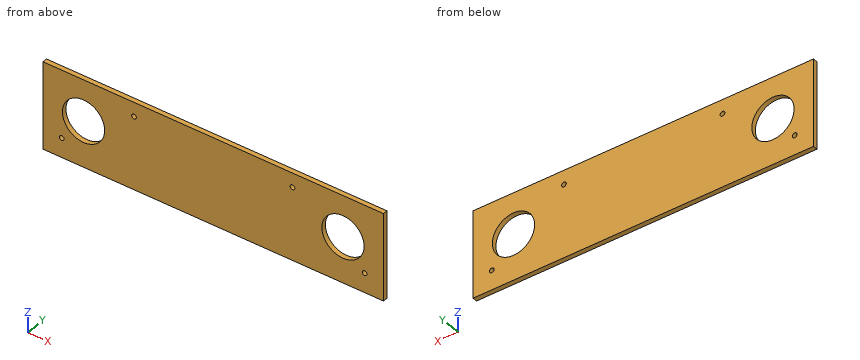
```python
from build123d import *

# Parameters (mm, degrees)
F0_W     = 145
F0_H     = 35
F1_DEPTH = 2
F2_R     = 1
F3_DEPTH = 25
F4_R     = 1
F5_DEPTH = 25
F6_R     = 9
F7_DEPTH = 25
F8_W     = 145
F8_H     = 2
F9_DEPTH = 2


with BuildPart() as f1:
    # F0 (on Front) → F1 (new body)
    with BuildSketch(Plane.XZ):
        Rectangle(F0_W, F0_H)
    extrude(amount=F1_DEPTH)

    # F2 (on face) → F3 (cut)
    with BuildSketch(Plane.XZ.offset(2)):
        with Locations((-33.75, 11.5)):
            Circle(F2_R)
        with Locations((33.75, 11.5)):
            Circle(F2_R)
    extrude(amount=-F3_DEPTH, mode=Mode.SUBTRACT)

    # F4 (on face) → F5 (cut)
    with BuildSketch(Plane.XZ.offset(2)):
        with Locations((-64.5, -11.25)):
            Circle(F4_R)
        with Locations((64.5, -11.25)):
            Circle(F4_R)
    extrude(amount=-F5_DEPTH, mode=Mode.SUBTRACT)

    # F6 (on face) → F7 (cut)
    with BuildSketch(Plane.XZ.offset(2)):
        with Locations((-55.25, 0)):
            Circle(F6_R)
        with Locations((55.25, 0)):
            Circle(F6_R)
    extrude(amount=-F7_DEPTH, mode=Mode.SUBTRACT)

    # F8 (on face) → F9 (join)
    with BuildSketch(Plane(origin=(0, 0, -17.5), x_dir=(1, 0, 0), z_dir=(0, 0, -1))):
        with Locations((0, 1)):
            Rectangle(F8_W, F8_H)
    extrude(amount=F9_DEPTH)


solid = f1.part
```
Could you check a few things on this model? Use its own coordinates, in mm. Round coordinates to 2 decimals unless told otherwise and drop trailing zeros. Order: outer loops, then holes, each group sorted by start corner. A loop starts at its lowest first (then second) coordinate and runs counter-clockwise, first axis right, second up. Notation, with made-up numbers: M -24,-32 L 34,-32 A32 cw 34,6 Z; hole C -31,-30 d9. An arc over 180 degrees is marked long. One line per question, with ' | ' between items. Start each with the question number.
(1) For P1, Ø14.5, axis at x = 55.25, z = 0, coming from the -Y side, with a flat end and sliding along its axis, tell me the tip position at first contact or that it passes through.
(2) Suppose I cut it at B-B on x = -55.25. List the corners of the cut face in (y, z) for me.
(3) Please list where these lines run through material, in increasing order: line 1 along Z through (x, y) = (64.5, -0.7); line 2 along Z through (x, y) = (55.25, -1.25); line 3 along X through (y, z) = (-1.5, -6).
(4) Suppose I cut it at A-A on y = -0.5. List the corners of the cut face in (x, z) for me, then the cut area to 3 significant figures.
Geometry results:
1) P1: through
2) outline: M -2,-19.5 L 0,-19.5 L 0,-9 L -2,-9 Z; M -2,9 L 0,9 L 0,17.5 L -2,17.5 Z
3) line 1: -19.5 to -12.25, -10.25 to 17.5 | line 2: -19.5 to -9, 9 to 17.5 | line 3: -72.5 to -61.96, -48.54 to 48.54, 61.96 to 72.5
4) outline: M -72.5,-19.5 L 72.5,-19.5 L 72.5,17.5 L -72.5,17.5 Z; hole C -64.5,-11.25 d2; hole C -55.25,0 d18; hole C -33.75,11.5 d2; hole C 33.75,11.5 d2; hole C 55.25,0 d18; hole C 64.5,-11.25 d2 | area: 4,840 mm²
